Could you check a few things on this model? Use its own coordinates, in mm. A direction names the side the tool comes from. Give positions to 0.01 mm unless a question says otherwise; leave off trailing zeros. Loops run counter-clockwise (first coordinate to the right, second up) from the corner with the lowest first, then second, coordinate; pieces in that order, holes last. Notation, with made-up numbers: M 80.5,-12.75 L 125.5,-12.75 A18 ccw 125.5,-8.75 Z; hole C 13.5,26.5 d6. An arc over 180 degrees is marked long. Return JSON: item names as keys, results as strings. Group by question number.
1. For faces 1 (the flat face through (11.5, 0, 2)), 2 (the flat face through (0, 8, 3)), which set-ups out of +Z, -Z, +X, -X, +Y, -Y let a thin tool reach every point of the face, with its end or its side?
2. If we section it at D-D (z = 1.35): Write out the boundary of the cut face in (x, y).
3. If we section it at A-A (x = 5): Write out the boundary of the cut face in (y, z).
4. If we section it at B-B (y = -3): Write out the boundary of the cut face in (x, z).
5. If we mould it in two halves opening along Y, with no side actions, what happens to faces 3 (the flat face through (-15, 0, 1)), 4 (the flat face through (0, 6.5, 2)), 5 (the flat face through (0, 16.5, 1))? For each: +Y half, -Y half, draft (parallel to the pull), parting line (faces both ways), or undercut.
6. If we section it at C-C (x = 0): Write out the boundary of the cut face in (y, z), plus the area to 3 significant figures.
7. Please list where these lines run through material, in increasing order: line 1 (Y direction, x = 0, z = 1.5); line 2 (X direction, y = 2.5, z = 0.3); line 3 (Y direction, x = -11.25, z = 1.4).
8. For pin 1 (3.5 mm diameter, centred on x = 0, y = 11.5, fed in from -Z), with a flat end and sliding along its axis, tell me the tip position at first contact or that it passes through.
```python
from build123d import *

# Parameters (mm, degrees)
SKETCH1_W           = 30
SKETCH1_H           = 33
BOSS_EXTRUDE1_DEPTH = 3
SKETCH2_W           = 23
SKETCH2_H           = 13
CUT_EXTRUDE1_DEPTH  = 23.5
SKETCH3_R           = 2
CUT_EXTRUDE2_DEPTH  = 3


with BuildPart() as part:
    # Sketch1 → Boss-Extrude1 (new body)
    with BuildSketch(Plane.XY):
        Rectangle(SKETCH1_W, SKETCH1_H)
    extrude(amount=BOSS_EXTRUDE1_DEPTH)

    # Sketch2 → Cut-Extrude1 (cut, through all)
    with BuildSketch(Plane.XY.offset(3)):
        Rectangle(SKETCH2_W, SKETCH2_H)
    extrude(amount=-CUT_EXTRUDE1_DEPTH, mode=Mode.SUBTRACT)

    # Sketch3 → Cut-Extrude2 (cut)
    with BuildSketch(Plane.XY.offset(3)):
        with Locations((0, 11.5)):
            Circle(SKETCH3_R)
        with Locations((0, -11.5)):
            Circle(SKETCH3_R)
    extrude(amount=-CUT_EXTRUDE2_DEPTH, mode=Mode.SUBTRACT)


solid = part.part
```
Answer:
{
 "1": {"face 1": "+Z, -Z", "face 2": "+Z, +X, -X, +Y, -Y"},
 "2": {"outline": "M -15,-16.5 L 15,-16.5 L 15,16.5 L -15,16.5 Z; hole M -11.5,-6.5 L 11.5,-6.5 L 11.5,6.5 L -11.5,6.5 Z; hole C 0,-11.5 d4; hole C 0,11.5 d4"},
 "3": {"outline": "M -16.5,0 L -6.5,0 L -6.5,3 L -16.5,3 Z; M 6.5,0 L 16.5,0 L 16.5,3 L 6.5,3 Z"},
 "4": {"outline": "M -15,0 L -11.5,0 L -11.5,3 L -15,3 Z; M 11.5,0 L 15,0 L 15,3 L 11.5,3 Z"},
 "5": {"face 3": "draft", "face 4": "undercut", "face 5": "+Y half"},
 "6": {"outline": "M -16.5,0 L -13.5,0 L -13.5,3 L -16.5,3 Z; M -9.5,0 L -6.5,0 L -6.5,3 L -9.5,3 Z; M 6.5,0 L 9.5,0 L 9.5,3 L 6.5,3 Z; M 13.5,0 L 16.5,0 L 16.5,3 L 13.5,3 Z", "area": "36.0 mm²"},
 "7": {"line 1": "y = -16.5 to -13.5, -9.5 to -6.5, 6.5 to 9.5, 13.5 to 16.5", "line 2": "x = -15 to -11.5, 11.5 to 15", "line 3": "y = -16.5 to -6.5, 6.5 to 16.5"},
 "8": {"pin 1": "passes through"}
}
